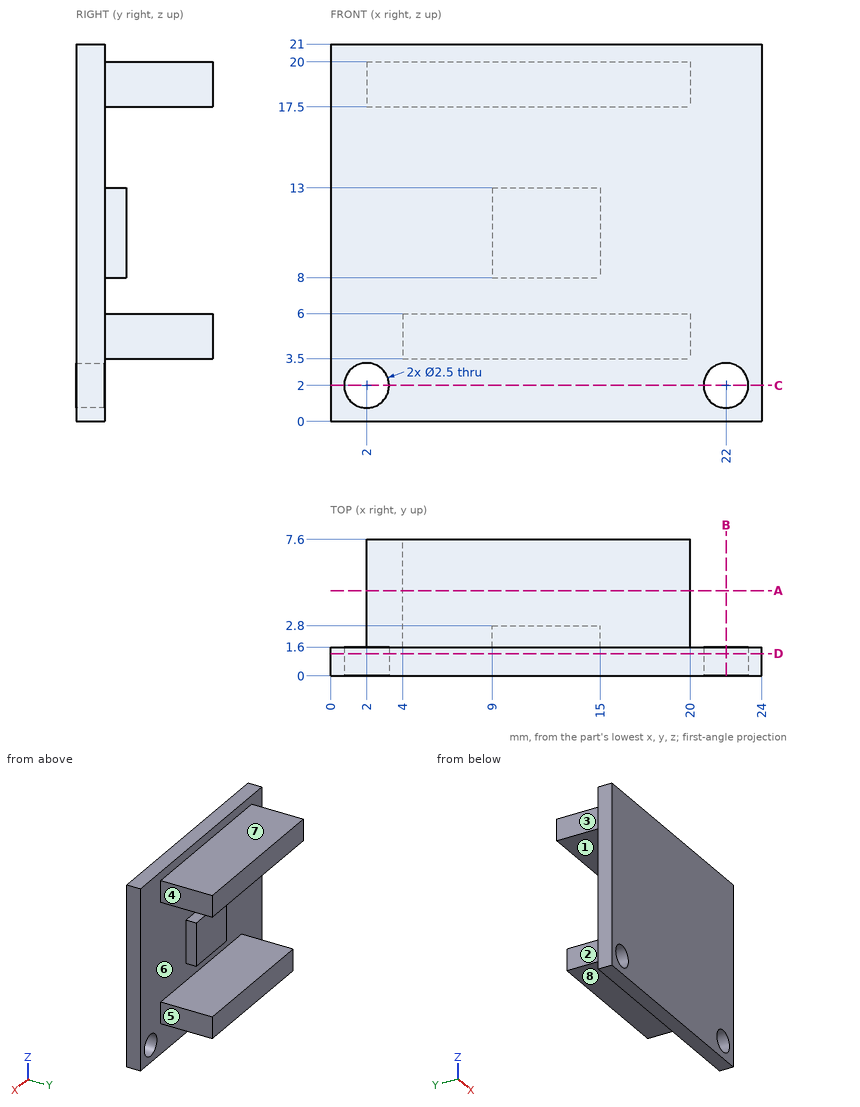
Geometry check sheet. Reference: drawing and pictorial views, mm from the part's lowest x, y, z. A direction names the side the tool comes from. Coordinates: 2 decimals unless noted, no trailing zeros. Write each loop counter-clockwise with the first axis right and the second up, starting at its lowest first coordinate (ties: lowest second). Pieces come first, ordered by that corner, then holes. Notation, with made-up numbers: (26.25, -11) -> (69.25, -11) arc R24 cw to (69.25, 15) -> close; hole circle Ø7 at (68, -7.75). An arc over 180 degrees is marked (long way). Use a Markdown table: item, result.
1. Release check for a two-part mould opening along Z. For the marked faces 5, 6, 7 and 8 record: pulls with the +Z half, pulls with the -Z half, needs draft (parallel to the pull), parting line crosses it, or undercut.
Reported:
| item | result |
|---|---|
| face 5 | needs draft |
| face 6 | undercut |
| face 7 | pulls with the +Z half |
| face 8 | pulls with the -Z half |
2. Scan lines: line 1 along X through (y, z) = (0.75, 2); line 2 along Z through (x, y) = (10.5, 5); line 3 along Z through (x, y) = (2, 0.75). Record each from-to range of solid material in increasing order.
Reported:
| item | result |
|---|---|
| line 1 | x = 0 to 0.75, 3.25 to 20.75, 23.25 to 24 |
| line 2 | z = 3.5 to 6, 17.5 to 20 |
| line 3 | z = 0 to 0.75, 3.25 to 21 |
3. Sectioned sample at A-A (y = 4.75). Enter the section's corners in (x, z).
Reported:
| item | result |
|---|---|
| outline | (2, 17.5) -> (20, 17.5) -> (20, 20) -> (2, 20) -> close; (4, 3.5) -> (20, 3.5) -> (20, 6) -> (4, 6) -> close |
4. Go/stop test with flat-tipped pins: pin 1 Ø1 at (x, y) = (12, 2.5) entering from -Z; pin 2 Ø0.8 at (y, z) = (5.5, 5) entering from +X; pin 3 Ø1.2 at (y, z) = (5, 18.5) entering from -X. Record where each tip stops, or that it passes through.
Reported:
| item | result |
|---|---|
| pin 1 | stops at z = 3.5 |
| pin 2 | stops at x = 20 |
| pin 3 | stops at x = 2 |
5. Sectioned sample at C-C (z = 2). Enter the section's corners in (x, y), plus the area to 3 significant figures.
Reported:
| item | result |
|---|---|
| outline | (0, 0) -> (0.75, 0) -> (0.75, 1.6) -> (0, 1.6) -> close; (3.25, 0) -> (20.75, 0) -> (20.75, 1.6) -> (3.25, 1.6) -> close; (23.25, 0) -> (24, 0) -> (24, 1.6) -> (23.25, 1.6) -> close |
| area | 30.4 mm2 |
6. Sectioned sample at B-B (x = 22). Enter the section's corners in (y, z).
Reported:
| item | result |
|---|---|
| outline | (0, 0) -> (1.6, 0) -> (1.6, 0.75) -> (0, 0.75) -> close; (0, 3.25) -> (1.6, 3.25) -> (1.6, 21) -> (0, 21) -> close |
7. Tool access check on the marked faces 1, 2, 3 and 4. Record the directions out of +Z, -Z, +X, -X, +Y, -Y that give a thin tool (end or side, any length) a straight path to the whole face; none if there is none.
Reported:
| item | result |
|---|---|
| face 1 | +X, -X, +Y |
| face 2 | -Z, -X, +Y |
| face 3 | +Z, -Z, -X, +Y |
| face 4 | +Z, -Z, +X, +Y |
8. Sectioned sample at D-D (y = 1.25). Enter the section's corners in (x, z), plus the area to 3 significant figures.
Reported:
| item | result |
|---|---|
| outline | (0, 0) -> (24, 0) -> (24, 21) -> (0, 21) -> close; hole circle Ø2.5 at (2, 2); hole circle Ø2.5 at (22, 2) |
| area | 494 mm2 |
